Check sheet for the drawn part. Datum: minimum x, y, z corner. Units: mm. Coordinates: 2 decimals unless noted, no trailing zeros. Loops run counter-clockwise (first coordinate to the right, second up) from the corner with the lowest first, then second, coordinate; pieces in that order, holes last. Notation, with made-up numbers: (75, -18) - (121, -18) arc R25 cw to (121, 9) - close; hole circle Ø5 at (59, -7.75). An arc over 180 degrees is marked (long way). Answer as CSV lines item,"result". Start each with the question number.
1. Gauge pin test, flat ends, axial feed: P1, Ø5, axis at y = 214, z = 966, coming from the -X side; P2, Ø4, axis at y = 121.5, z = 269.5, coming from the -X side; P3, Ø1.5, axis at x = 73, z = 1380, coming from the -Y side. Record the tip position at first contact, or that the pin passes through.
2. Cross-section at B-B (y = 248.5). Enter the section's corners in (x, z).
3. Cross-section at A-A (x = 110). Enter the section's corners in (y, z).
4. Cross-section at D-D (y = 172). Enter the section's corners in (x, z), plus the area to 3 significant figures.
5. Material ranges on line 1 (Z direction, x = 95.5, y = 231); line 2 (Y direction, x = 113, z = 922); line 3 (Y direction, x = 104.5, z = 529), recorded low to high. Write a range as [from, to].
6. Cross-section at C-C (z = 950). Enter the section's corners in (x, y).
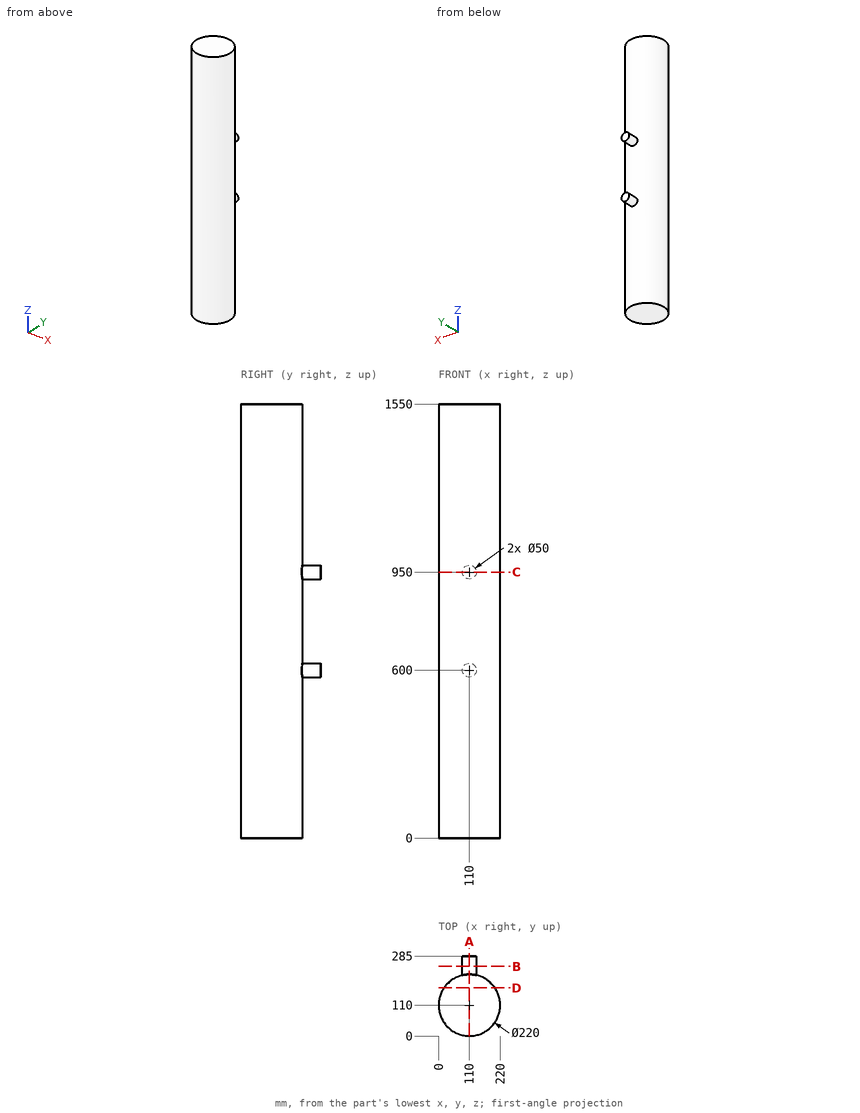
Values follow:
1,P1,"stops at x = 67.6"
1,P2,"stops at x = 0.41"
1,P3,"stops at y = 6.14"
2,outline,"circle Ø50 at (110, 600); circle Ø50 at (110, 950)"
3,outline,"(0, 0) - (220, 0) - (220, 575) - (285, 575) - (285, 625) - (220, 625) - (220, 925) - (285, 925) - (285, 975) - (220, 975) - (220, 1550) - (0, 1550) - close"
4,outline,"(19.14, 0) - (200.86, 0) - (200.86, 1550) - (19.14, 1550) - close"
4,area,"282,000 mm²"
5,line 1,"z = [579.63, 620.37], [929.63, 970.37]"
5,line 2,"y = [0.04, 219.96]"
5,line 3,"y = [0.14, 219.86]"
6,outline,"(85, 217.12) arc R110 ccw (long way) to (135, 217.12) - (135, 285) - (85, 285) - close"
